Autodesk Inventor part; units mm, degrees
ref_plane "YZ Plane" through (0, 0, 0) normal (1, 0, 0) x (0, 1, 0)
ref_plane "XZ Plane" through (0, 0, 0) normal (0, 1, 0) x (-1, 0, 0)
ref_plane "XY Plane" through (0, 0, 0) normal (0, 0, 1) x (1, 0, 0)
sketch "Sketch1" plane through (0, 0, 0) normal (1, 0, 0) x (0, 1, 0)
  line L0 (0, 0) -> (0, 7.75) construction
  line L1 (0, 7.75) -> (6.7117, 3.875)
  line L2 (6.7117, 3.875) -> (6.7117, -3.875)
  line L3 (6.7117, -3.875) -> (0, -7.75)
  line L4 (0, -7.75) -> (-6.7117, -3.875)
  line L5 (-6.7117, -3.875) -> (-6.7117, 3.875)
  line L6 (-6.7117, 3.875) -> (0, 7.75)
  dimension "d0" = 7.75
extrude "Extrusion1" add sketch "Sketch1" along normal blind 10
sketch "Sketch2" plane through (10, 0, 0) normal (1, 0, 0) x (0, 0, -1)
  circle A0 centre (0, 0) radius 10
  dimension "d3" = 20
extrude "Extrusion2" add sketch "Sketch2" along normal blind 3
sketch "Sketch3" plane through (13, 0, 0) normal (1, 0, 0) x (0, 0, -1)
  circle A0 centre (0, 0) radius 3.625
  dimension "d6" = 7.25
extrude "Extrusion3" cut sketch "Sketch3" against normal blind 15
properties part number "smallHub 9-25"
Read the model definition and answer for the solid it produces. Units are mm, in the model's axes. A direction names the side the tool comes from. Give positions to 0.01 mm unless a question says otherwise; leave off trailing zeros. Write each loop counter-clockwise with the first axis right and the second up, starting at its lowest first coordinate (ties: lowest second). Pieces come first, ordered by that corner, then holes. Notation, with made-up numbers: (-19.75, 28.5) - (37.25, 28.5) arc R20 cw to (37.25, 62.5) - close; hole circle Ø4 at (7.5, 81.25). An arc over 180 degrees is marked (long way). Return JSON: item names as keys, results as strings.
Q1. A cutting plane is placed at C-C, the plane y = 1. Determine the outline of the cut face in (x, z).
Reply:
{"outline": "(0, -7.17) - (10, -7.17) - (10, -9.95) - (13, -9.95) - (13, -3.48) - (0, -3.48) - close; (0, 3.48) - (13, 3.48) - (13, 9.95) - (10, 9.95) - (10, 7.17) - (0, 7.17) - close"}
Q2. For a pull along Y with two mould halves and no side action, classify faces 6 (the face through (11.48, 9.76, 2.17)), 7 (the face through (6.6, -3.2, -1.7)), 8 (the face through (5, 6.712, 0)), 9 (the face through (4.93, -3.31, -5.84)) as released by +Y, released by -Y, zero draft, split by the parting line, or undercut.
Reply:
{"face 6": "split by the parting line", "face 7": "undercut", "face 8": "released by +Y", "face 9": "released by -Y"}
Q3. A cutting plane is placed at D-D, the plane z = -7. Determine the outline of the cut face in (x, y), and give its area (3 significant figures).
Reply:
{"outline": "(0, -1.3) - (10, -1.3) - (10, -7.14) - (13, -7.14) - (13, 7.14) - (10, 7.14) - (10, 1.3) - (0, 1.3) - close", "area": "68.8 mm²"}
Q4. A cutting plane is placed at A-A, the plane z = 0. Determine the outline of the cut face in (x, y) (3 decimals), and give its area (4 significant figures).
Reply:
{"outline": "(0, -6.712) - (10, -6.712) - (10, -10) - (13, -10) - (13, -3.625) - (0, -3.625) - close; (0, 3.625) - (13, 3.625) - (13, 10) - (10, 10) - (10, 6.712) - (0, 6.712) - close", "area": "100.0 mm²"}
Q5. For faces 1 (the face through (4.93, 3.403, -5.785)), 2 (the face through (4.93, 3.31, 5.84)), 3 (the face through (4.93, -3.403, 5.785)), 4 (the face through (5, -6.712, 0)), 5 (the face through (10, 7, 0)), determine the directions among +Z, -Z, +X, -X, +Y, -Y from which every point of the face is accessible in a straight line to the end or side of a thin tool.
Reply:
{"face 1": "-Z, -X, +Y", "face 2": "+Z, -X, +Y", "face 3": "+Z, -X, -Y", "face 4": "+Z, -Z, -X, -Y", "face 5": "-X"}
Q6. Given P1, Ø1.5, axis at x = 9.5, y = -6, coming from the -Z side; P2, Ø2, axis at x = 9.5, z = 7, coming from the +Y side; P3, Ø6, axis at x = 3.5, z = -3.5, coming from the -Y side; P4, Ø8.5, axis at y = 0, z = 0, coming from the -X side, each flat-ended and moving along its own axis, determine where each tip first touches the part or whether it passes through.
Reply:
{"P1": "z = -8.39", "P2": "y = 7.9", "P3": "y = -6.71", "P4": "x = 0"}
Q7. A cutting plane is placed at B-B, the plane x = 4.25. Determine the outline of the cut face in (y, z) (3 decimals), and give its area (3 significant figures).
Reply:
{"outline": "(-6.712, -3.875) - (0, -7.75) - (6.712, -3.875) - (6.712, 3.875) - (0, 7.75) - (-6.712, 3.875) - close; hole circle Ø7.25 at (0, 0)", "area": "115 mm²"}
Q8. Consider line 1 along Y through (x, z) = (8, 0) (3 decimals); line 2 along X through (y, z) = (-7.5, -2); line 3 along Z through (x, y) = (5.5, 1). Determine where each line is inside the solid, lowest interval first. Write a range as [from, to].
Reply:
{"line 1": "[-6.712, -3.625], [3.625, 6.712]", "line 2": "[10, 13]", "line 3": "[-7.17, -3.48], [3.48, 7.17]"}
